from build123d import *

# Parameters (mm, degrees)
F1_DEPTH = 8.5
F3_DEPTH = 8.501
F5_DEPTH = 8.501
F6_R     = 13.49999
F7_SIZE2 = 5.1961524227
F7_SIZE  = 3


# Not quite as in the source:
# - a fillet or chamfer is up to 0.001 mm smaller than in the source, because OpenCascade refuses the exact size


with BuildPart() as f1:
    # F0 (on Top) → F1 (new body)
    with BuildSketch(Plane.XY):
        with BuildLine():
            Line((-298.5, -23.5), (298.5, -23.5))
            ThreePointArc((298.5, -23.5), (308.045941546, -19.545941546), (312, -10))
            Line((312, -10), (312, 10))
            ThreePointArc((312, 10), (308.045941546, 19.545941546), (298.5, 23.5))
            Line((298.5, 23.5), (-298.5, 23.5))
            ThreePointArc((-298.5, 23.5), (-308.045941546, 19.545941546), (-312, 10))
            Line((-312, 10), (-312, -10))
            ThreePointArc((-312, -10), (-308.045941546, -19.545941546), (-298.5, -23.5))
        make_face()
    extrude(amount=F1_DEPTH)

    # F2 (on face) → F3 (cut, through all)
    with BuildSketch(Plane.XY.offset(8.5)):
        with BuildLine():
            Line((-13.5, 3.5), (13.5, 3.5))
            ThreePointArc((13.5, 3.5), (18.0961940777, 5.4038059223), (20, 10))
            Line((20, 10), (20, 23.5))
            Line((20, 23.5), (-20, 23.5))
            Line((-20, 23.5), (-20, 10))
            ThreePointArc((-20, 10), (-18.0961940777, 5.4038059223), (-13.5, 3.5))
        make_face()
    extrude(amount=-F3_DEPTH, mode=Mode.SUBTRACT)

    # F4 (on face) → F5 (cut, through all)
    with BuildSketch(Plane.XY.offset(8.5)):
        with BuildLine():
            Line((-308.5, 10), (-308.5, -10))
            ThreePointArc((-308.5, -10), (-305.5710678119, -17.0710678119), (-298.5, -20))
            Line((-298.5, -20), (298.5, -20))
            ThreePointArc((298.5, -20), (305.5710678119, -17.0710678119), (308.5, -10))
            Line((308.5, -10), (308.5, 10))
            ThreePointArc((308.5, 10), (305.5710678119, 17.0710678119), (298.5, 20))
            Line((298.5, 20), (33.5, 20))
            ThreePointArc((33.5, 20), (26.4289321881, 17.0710678119), (23.5, 10))
            ThreePointArc((23.5, 10), (20.5710678119, 2.9289321881), (13.5, 0))
            Line((13.5, 0), (-13.5, 0))
            ThreePointArc((-13.5, 0), (-20.5710678119, 2.9289321881), (-23.5, 10))
            ThreePointArc((-23.5, 10), (-26.4289321881, 17.0710678119), (-33.5, 20))
            Line((-33.5, 20), (-298.5, 20))
            ThreePointArc((-298.5, 20), (-305.5710678119, 17.0710678119), (-308.5, 10))
        make_face()
    extrude(amount=-F5_DEPTH, mode=Mode.SUBTRACT)

    # F6 (radius 13.5 in the source; OpenCascade refuses exactly that, so slightly less here)
    f6_edges = [f1.edges().sort_by_distance(p)[0] for p in [
        (-20, 23.5, 4.25),
        (20, 23.5, 4.25),
    ]]
    fillet(f6_edges, radius=F6_R)

    # F7
    f7_edges = [f1.edges().sort_by_distance(p)[0] for p in [
        (165.999995, 23.5, 8.5),
    ]]
    f7_side = f1.faces().sort_by_distance((-165.999995, 22.874232, 8.5))[0]
    chamfer(f7_edges, length=F7_SIZE, length2=F7_SIZE2, reference=f7_side)


solid = f1.part
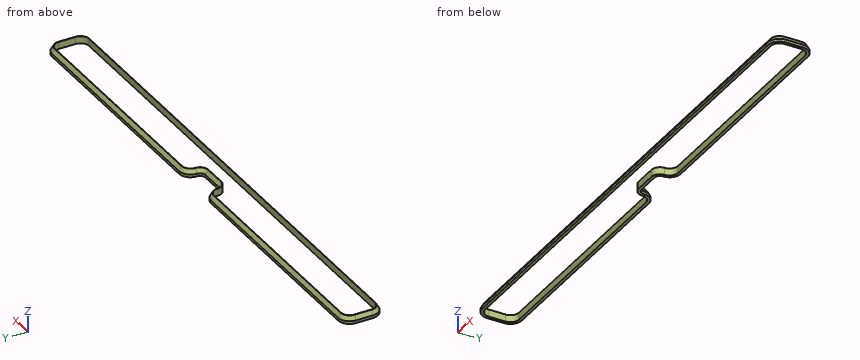
Geometry check sheet. Reference: the model listing, model coordinates, mm. Give positions to 0.01 mm unless a question says otherwise; leave off trailing zeros. Loops run counter-clockwise (first coordinate to the right, second up) from the corner with the lowest first, then second, coordinate; pieces in that order, holes last. Notation, with made-up numbers: M -40,15 L -23,15 A15 ccw -23,38 Z; hole C 59.5,12.25 d10. An arc over 180 degrees is marked long. Answer as a JSON object with one key per item and string values. Group by question number.
Item 1: Gauge pin test, flat ends, axial feed: pin 1 (1 mm diameter, centred on x = 1, z = 2.5, fed in from +Y); pin 2 (4 mm diameter, centred on y = -3, z = 6, fed in from -X); pin 3 (1 mm diameter, centred on x = -40, z = 6.5, fed in from -Y). Record the tip position at first contact, or that the pin passes through.
Item 2: Material ranges on L1, parallel to X at y = -6, z = 3.25; L2, parallel to Y at x = 266, z = 3; L3, parallel to X at y = 15.5, z = 2.25, recorded low to high.
Item 3: Sectioned sample at A-A on x = -0.5. Record the boundary of the cut face in (y, z), plus the area to 3 significant figures.
Findings below:
{
 "1": {"pin 1": "y = 3.5", "pin 2": "x = -311.6", "pin 3": "y = -21.94"},
 "2": {"L1": "-312 to -308.5, 308.5 to 312", "L2": "-23.5 to -20, 20 to 23.5", "L3": "-310.83 to -306.85, -25.15 to -21.17, 21.17 to 25.15, 306.85 to 310.83"},
 "3": {"outline": "M -23.5,0 L -20,0 L -20,8.5 L -20.5,8.5 L -23.5,3.3 Z; M 0,0 L 3.5,0 L 3.5,3.3 L 0.5,8.5 L 0,8.5 Z", "area": "43.9 mm2"}
}
